Here's how the part is built. I have some questions about the finished solid (model axes, mm). A direction names the side the tool comes from. Round coordinates to 2 decimals unless told otherwise and drop trailing zeros. Loops run counter-clockwise (first coordinate to the right, second up) from the corner with the lowest first, then second, coordinate; pieces in that order, holes last. Notation, with made-up numbers: M 51.5,-4 L 81.5,-4 A35 ccw 81.5,35 Z; hole C 24,61 d7. An arc over 180 degrees is marked long. Put each result on its own line as item: value. Start each with the question number.
```python
from build123d import *

# Parameters (mm, degrees)
SKETCH1_W           = 6
SKETCH1_H           = 6
BOSS_EXTRUDE1_DEPTH = 5
SKETCH2_W           = 6
SKETCH2_H           = 1
CUT_EXTRUDE1_DEPTH  = 2
CUT_EXTRUDE2_DEPTH  = 2
CUT_EXTRUDE3_DEPTH  = 2


with BuildPart() as part:
    # Sketch1 → Boss-Extrude1 (new body)
    with BuildSketch(Plane(origin=(0, 0, 0), x_dir=(1, 0, 0), z_dir=(0, 1, 0))):
        Rectangle(SKETCH1_W, SKETCH1_H)
    extrude(amount=BOSS_EXTRUDE1_DEPTH)

    # Sketch2 → Cut-Extrude1 (cut)
    with BuildSketch(Plane.ZY.offset(3)):
        Polygon((3, 5), (-3, 5), (3, 3), align=None)
        with Locations((0, 0.5)):
            Rectangle(SKETCH2_W, SKETCH2_H)
    extrude(amount=-CUT_EXTRUDE1_DEPTH, mode=Mode.SUBTRACT)

    # Sketch3 → Cut-Extrude2 (cut)
    with BuildSketch(Plane.ZY.offset(1)):
        Polygon((-3, 5), (-3, 4), (3, 2), (3, 3), align=None)
        Polygon((3, 3), (3, 5), (-3, 5), align=None)
    extrude(amount=-CUT_EXTRUDE2_DEPTH, mode=Mode.SUBTRACT)

    # Sketch4 → Cut-Extrude3 (cut)
    with BuildSketch(Plane.ZY.offset(-1)):
        Polygon((-3, 5), (3, 2), (3, 5), align=None)
    extrude(amount=-CUT_EXTRUDE3_DEPTH, mode=Mode.SUBTRACT)


solid = part.part
```
1) Suppose I cut it at B-B (z = -1.5). Write out the boundary of the cut face in (x, y).
2) On a 3-axis mill with a long thin cutter (end or side, diameter ignored), from which of +Z, -Z, +X, -X, +Y, -Y can I reach the whole of each face in a straight line? I mean faces 5 (the face through (-2, 1, 0)), 6 (the face through (-2, 4, 0)), 7 (the face through (0, 3, 0)), 8 (the face through (2, 3.5, 0)). Say none if no direction works.
3) Suppose I cut it at C-C (y = 3.65). Write out the boundary of the cut face in (x, z), plus the area to 3 significant figures.
4) If I drill on probe 1 along X at (y, z) = (3.7, -1.5); probe 2 along X at (y, z) = (0.3, -1); probe 3 along X at (y, z) = (3.2, 1.5), over which ranges is the centre line in solid material (lowest first)? Write a range as from..to.
5) Suppose I cut it at D-D (x = 1.8). Write out the boundary of the cut face in (y, z).
6) Suppose I cut it at A-A (y = 2.65). Write out the boundary of the cut face in (x, z), plus the area to 3 significant figures.
7) I'm going to push flat-ended pins straight in: P1, Ø1.5, axis at x = -0.5, z = 1, coming from the +Y side; P2, Ø1, axis at x = -2, z = 1, coming from the -Y side; P3, Ø2, axis at y = 4.5, z = 1.5, coming from the +X side. Where does each tip first touch, or does it pass through?
8) If we mould it in two halves opening along X, with no side actions, what happens to faces 1 (the face through (0, 2, -3)), 2 (the face through (3, 2, -1)), 3 (the face through (-1, 3.6, 0)), 4 (the face through (-3, 3, 0))? For each: pulls with the +X half, pulls with the -X half, needs draft (parallel to the pull), parting line crosses it, or undercut.
Results are:
1. outline: M -3,1 L -1,1 L -1,0 L 3,0 L 3,4.25 L 1,4.25 L 1,3.5 L -1,3.5 L -1,4.5 L -3,4.5 Z
2. face 5: +Z, -Z, -X, -Y
2. face 6: +Z, +X, -X, +Y
2. face 7: +Z, +Y
2. face 8: +Z, +X, +Y
3. outline: M -3,-3 L 3,-3 L 3,-0.3 L 1,-0.3 L 1,-1.95 L -1,-1.95 L -1,1.05 L -3,1.05 Z
3. area: 15.6 mm²
4. probe 1: -3..-1, 1..3
4. probe 2: -1..3
4. probe 3: -3..-1
5. outline: M 0,-3 L 5,-3 L 2,3 L 0,3 Z
6. outline: M -3,-3 L 3,-3 L 3,1.7 L 1,1.7 L 1,1.05 L -1,1.05 L -1,3 L -3,3 Z
6. area: 29.5 mm²
7. P1: y = 3.85
7. P2: y = 1
7. P3: x = -1
8. face 1: needs draft
8. face 2: pulls with the +X half
8. face 3: undercut
8. face 4: pulls with the -X half
